```python
from build123d import *

# Parameters (mm, degrees)
SALIENTE_EXTRUIR2_DEPTH = 15
CROQUIS3_R              = 1.55
SALIENTE_EXTRUIR3_DEPTH = 2


with BuildPart() as part:
    # Croquis2 → Saliente-Extruir2 (new body)
    with BuildSketch(Plane.XY):
        with BuildLine():
            Line((2.8, -5.306599665), (2.8, -5.5))
            Line((2.8, -5.5), (2, -5.5))
            Line((2, -5.5), (2, -4.582575695))
            ThreePointArc((2, -4.582575695), (0, 5), (-2, -4.582575695))
            Line((-2, -4.582575695), (-2, -5.5))
            Line((-2, -5.5), (-2.8, -5.5))
            Line((-2.8, -5.5), (-2.8, -5.306599665))
            ThreePointArc((-2.8, -5.306599665), (0, 6), (2.8, -5.306599665))
        make_face()
    extrude(amount=SALIENTE_EXTRUIR2_DEPTH)

    # Croquis3 → Saliente-Extruir3 (add)
    # profile 1 of 2: a face of its own
    with BuildSketch(Plane.XZ.offset(5.5)):
        with BuildLine():
            Line((2, 0), (2, 15))
            Line((2, 15), (11.1, 15))
            ThreePointArc((11.1, 15), (13.079898987, 14.179898987), (13.9, 12.2))
            Line((13.9, 12.2), (13.9, 2.8))
            ThreePointArc((13.9, 2.8), (13.079898987, 0.820101013), (11.1, 0))
            Line((11.1, 0), (2, 0))
        make_face()
        with Locations(Location((11.1, 2.35, 0), (0, 0, 270))):
            Circle(CROQUIS3_R, mode=Mode.SUBTRACT)
    # profile 2 of 2: a face of its own
    with BuildSketch(Plane.XZ.offset(5.5)):
        with BuildLine():
            Line((-13.9, 2.8), (-13.9, 12.2))
            ThreePointArc((-13.9, 12.2), (-13.079898987, 14.179898987), (-11.1, 15))
            Line((-11.1, 15), (-2, 15))
            Line((-2, 15), (-2, 0))
            Line((-2, 0), (-11.1, 0))
            ThreePointArc((-11.1, 0), (-13.079898987, 0.820101013), (-13.9, 2.8))
        make_face()
        with Locations(Location((-11.1, 12.65, 0), (0, 0, 270))):
            Circle(CROQUIS3_R, mode=Mode.SUBTRACT)
    extrude(amount=SALIENTE_EXTRUIR3_DEPTH)


solid = part.part
```
The model under review builds one solid part; all positions refer to its coordinate system, in mm. A direction names the side the tool comes from. Round coordinates to 2 decimals unless told otherwise and drop trailing zeros. Order: outer loops, then holes, each group sorted by start corner. A loop starts at its lowest first (then second) coordinate and runs counter-clockwise, first axis right, second up.
(1) For P1, Ø8, axis at x = 0.5, y = 3.5, coming from the +Z side; P2, Ø5, axis at x = 11.1, z = 2.35, coming from the +Y side, all flat-tipped, find the tip position at first contact; note any pin that passes through.
Working result:
P1: stops at z = 15
P2: stops at y = -5.5
(2) Take a section at D-D, the plane z = 2.35. State the section outline as (x, y) points, plus the area to 3 significant figures.
Working result:
outline: (-13.86, -7.5) - (-2, -7.5) - (-2, -4.58) arc R5 cw (long way) to (2, -4.58) - (2, -7.5) - (9.55, -7.5) - (9.55, -5.5) - (2.8, -5.5) - (2.8, -5.31) arc R6 ccw (long way) to (-2.8, -5.31) - (-2.8, -5.5) - (-13.86, -5.5) - close; (12.65, -7.5) - (13.86, -7.5) - (13.86, -5.5) - (12.65, -5.5) - close
area: 71.7 mm2
(3) Take a section at A-A, the plane y = 0. State the section outline as (x, z) points, plus the area to 3 significant figures.
Working result:
outline: (-6, 0) - (-5, 0) - (-5, 15) - (-6, 15) - close; (5, 0) - (6, 0) - (6, 15) - (5, 15) - close
area: 30.0 mm2
(4) Wall thickness on L1, parallel to X at y = -6.5, z = 7; L2, parallel to X at y = 0, z = 10.25; L3, parallel to X at y = -6.3, z = 12.65: over which ranges is each line inside the solid? List them lowest first.
Working result:
L1: x = -13.9 to -2, 2 to 13.9
L2: x = -6 to -5, 5 to 6
L3: x = -13.86 to -12.65, -9.55 to -2, 2 to 13.86
(5) Tool access review of faces 5 (the face through (8, -5.5, 8)), 6 (the face through (-2, -6, 7)), 7 (the face through (-8, -5.5, 8)): name each direction out of +Z, -Z, +X, -X, +Y, -Y from which nothing blocks a thin tool from reaching the whole face with its end or side.
Working result:
face 5: +Z, -Z, +X
face 6: +Z, -Z, -Y
face 7: +Z, -Z, -X
(6) Take a section at C-C, the plane x = -5.5. State the section outline as (y, z) points, plus the area to 3 significant figures.
Working result:
outline: (-7.5, 0) - (-5.5, 0) - (-5.5, 15) - (-7.5, 15) - close; (-2.4, 0) - (2.4, 0) - (2.4, 15) - (-2.4, 15) - close
area: 102 mm2
(7) Mouldability with a two-part tool opening along X and no side actions: class faces 1 (the face through (0, 5, 7)), 2 (the face through (2, -6, 7)), 3 (the face through (13.1, -6.49, 0.84)), 4 (the face through (3, -5, 0)) as released by +X, released by -X, zero draft, split by the parting line, or undercut.
Working result:
face 1: undercut
face 2: undercut
face 3: released by +X
face 4: zero draft
(8) Take a section at B-B, the plane z = 9. State the section outline as (x, y) points, plus the area to 3 significant figures.
Working result:
outline: (-13.9, -7.5) - (-2, -7.5) - (-2, -4.58) arc R5 cw (long way) to (2, -4.58) - (2, -7.5) - (13.9, -7.5) - (13.9, -5.5) - (2.8, -5.5) - (2.8, -5.31) arc R6 ccw (long way) to (-2.8, -5.31) - (-2.8, -5.5) - (-13.9, -5.5) - close
area: 78.1 mm2
